Design review of the part built by this model. Coordinates are the model's own, in mm. A direction names the side the tool comes from. Coordinates: 2 decimals unless noted, no trailing zeros. Loops run counter-clockwise (first coordinate to the right, second up) from the corner with the lowest first, then second, coordinate; pieces in that order, holes last. Notation, with made-up numbers: M -15,-19.75 L 27,-19.75 A29 cw 27,1.25 Z; hole C 40,-29.75 d1. An arc over 180 degrees is marked long. Answer as CSV lines item,"result". Start each with the question number.
from build123d import *

# Parameters (mm, degrees)
BOSS_EXTRUDE1_DEPTH = 3
SKETCH3_R           = 6
BOSS_EXTRUDE2_DEPTH = 4
SKETCH4_R           = 9
BOSS_EXTRUDE3_DEPTH = 25.5
SKETCH5_R           = 6.5
BOSS_EXTRUDE4_DEPTH = 19
SKETCH6_R           = 2.5
BOSS_EXTRUDE5_DEPTH = 13
SKETCH8_R           = 5.5
BOSS_EXTRUDE6_DEPTH = 29
SKETCH9_R           = 5.5
BOSS_EXTRUDE7_DEPTH = 34
BOSS_EXTRUDE7_TAPER = 3
SKETCH10_R          = 3
BOSS_EXTRUDE8_DEPTH = 40


with BuildPart() as part:
    # Sketch2 → Boss-Extrude1 (new body)
    with BuildSketch(Plane(origin=(-50, 0, 0), x_dir=(0, 0, -1), z_dir=(1, 0, 0))):
        Polygon((-5.051814855, 8.75), (-10.103629711, 0), (-5.051814855, -8.75), (5.051814855, -8.75), (10.103629711, 0), (5.051814855, 8.75), align=None)
    extrude(amount=BOSS_EXTRUDE1_DEPTH)

    # Sketch3 → Boss-Extrude2 (add)
    with BuildSketch(Plane(origin=(-47, 0, 0), x_dir=(0, 0, -1), z_dir=(1, 0, 0))):
        Circle(SKETCH3_R)
    extrude(amount=BOSS_EXTRUDE2_DEPTH)

    # Sketch4 → Boss-Extrude3 (add)
    with BuildSketch(Plane(origin=(-43, 0, 0), x_dir=(0, 0, -1), z_dir=(1, 0, 0))):
        Circle(SKETCH4_R)
    extrude(amount=BOSS_EXTRUDE3_DEPTH)

    # Sketch5 → Boss-Extrude4 (add)
    with BuildSketch(Plane(origin=(-17.5, 0, 0), x_dir=(0, 0, -1), z_dir=(1, 0, 0))):
        Circle(SKETCH5_R)
    extrude(amount=BOSS_EXTRUDE4_DEPTH)

    # Sketch6 → Boss-Extrude5 (add)
    with BuildSketch(Plane.ZY.offset(50)):
        with Locations(Location((0, 0, 0), (0, 0, 180))):
            Circle(SKETCH6_R)
    extrude(amount=BOSS_EXTRUDE5_DEPTH)

    # Sketch8 → Boss-Extrude6 (add)
    with BuildSketch(Plane(origin=(1.125, 0.649519053, 0), x_dir=(0, 0, -1), z_dir=(0.8660254037844379, 0.5000000000000012, 0))):
        with Locations(Location((0, 0, 0), (0, 0, 187.837479763))):
            Circle(SKETCH8_R)
    extrude(amount=BOSS_EXTRUDE6_DEPTH)

    # Sketch9 → Boss-Extrude7 (add)
    with BuildSketch(Plane(origin=(26.23973671, 15.149519053, 0), x_dir=(0, 0, -1), z_dir=(0.8660254037844379, 0.5000000000000012, 0))):
        with Locations(Location((0, 0, 0), (0, 0, 187.837479763))):
            Circle(SKETCH9_R)
    extrude(amount=BOSS_EXTRUDE7_DEPTH, taper=BOSS_EXTRUDE7_TAPER)

    # Sketch10 → Boss-Extrude8 (add)
    with BuildSketch(Plane(origin=(55.684600438, 32.149519053, 0), x_dir=(0, 0, -1), z_dir=(0.8660254037844379, 0.5000000000000012, 0))):
        with Locations(Location((0, 0, 0), (0, 0, 90))):
            Circle(SKETCH10_R)
    extrude(amount=BOSS_EXTRUDE8_DEPTH)


solid = part.part
Item 1: For faces 1 (the face through (-8.133, -6.345, 1.409)), 2 (the face through (-49, -8.75, 0)), 3 (the face through (-48.521, -4.314, 7.613)), 4 (the face through (-50, 2, -2)), list the 3-axis set-ups (+Z, -Z, +X, -X, +Y, -Y) from which the entire face can be reached by the end or side of a thin tool; tool diameter is ignored.
Item 2: For line 1 along Z through (x, y) = (17, 14.5); line 2 along Y through (x, z) = (-12, -2); line 3 along X through (y, z) = (46, -1.5), list the stretches that pass through material, from the lowest coordinate up. Write a range as from..to.
Item 3: Add section A-A (x = -53). Give the boundary of the cut face in (y, z), plus the area to 3 significant figures.
Item 4: For pin 1 (9 mm diameter, centred on y = 4, z = -0.5, fed in from +X); pin 2 (10 mm diameter, centred on x = 72, z = -3, fed in from +Y); pin 3 (2.5 mm diameter, centred on x = -48.5, z = -2, fed in from -Y), all flat-tipped, find the tip position at first contact; note any pin that passes through.
Item 5: Add section C-C (x = -8). Give the boundary of the cut face in (y, z).
Item 6: Mouldability with a two-part tool opening along X and no side actions: class faces 5 (the face through (-47, 6, -2)), 6 (the face through (-48.52, -4.44, -7.54)), 7 (the face through (42.476, 21.503, -3.78)) as released by +X, released by -X, zero draft, split by the parting line, or undercut.
Response:
1,face 1,"none"
1,face 2,"+Z, -Z, -X, -Y"
1,face 3,"+Z, -X, -Y"
1,face 4,"-X"
2,line 1,"-3.71..3.71"
2,line 2,"-6.18..6.18"
2,line 3,"74.48..84.87"
3,outline,"C 0,0 d5"
3,area,"19.6 mm²"
4,pin 1,"x = 25.7"
4,pin 2,"y = 47.5"
4,pin 3,"y = -8.75"
5,outline,"C 0,0 d13"
6,face 5,"undercut"
6,face 6,"zero draft"
6,face 7,"split by the parting line"
